Source: CAD feature listing. Evaluate the final solid. Frame: model axes, mm. Face numbers are marked on the shaded views. Give positions to 0.01 mm unless a question says otherwise; leave off trailing zeros. Loops run counter-clockwise (first coordinate to the right, second up) from the corner with the lowest first, then second, coordinate; pieces in that order, holes last.
from build123d import *

# Parameters (mm, degrees)
SKETCH_1_R          = 28
SKETCH_1_R_2        = 2.15
SKETCH_1_R_3        = 15
EXTRUDE_1_DEPTH     = 5
CUT_EXTRUDE_3_DEPTH = 1
SKETCH_5_R          = 5
CUT_EXTRUDE_5_DEPTH = 2
SKETCH_6_R          = 4.5
CUT_EXTRUDE_6_DEPTH = 1


with BuildPart() as part:
    # 草图1 → 凸台-拉伸1 (new body)
    with BuildSketch(Plane(origin=(0, 0, 0), x_dir=(1, 0, 0), z_dir=(0, 1, 0))):
        Circle(SKETCH_1_R)
        with Locations((13.980630511, -16.661466638)):
            Circle(SKETCH_1_R_2, mode=Mode.SUBTRACT)
        with Locations((13.980630511, 16.661466638)):
            Circle(SKETCH_1_R_2, mode=Mode.SUBTRACT)
        with Locations((21.75, 0)):
            Circle(SKETCH_1_R_2, mode=Mode.SUBTRACT)
        with Locations((-13.980630511, -16.661466638)):
            Circle(SKETCH_1_R_2, mode=Mode.SUBTRACT)
        with Locations((-21.75, 0)):
            Circle(SKETCH_1_R_2, mode=Mode.SUBTRACT)
        with Locations((-13.980630511, 16.661466638)):
            Circle(SKETCH_1_R_2, mode=Mode.SUBTRACT)
        Circle(SKETCH_1_R_3, mode=Mode.SUBTRACT)
    extrude(amount=EXTRUDE_1_DEPTH)

    # 草图2 → 切除-拉伸3 (cut)
    with BuildSketch(Plane(origin=(0, 0, 0), x_dir=(1, 0, 0), z_dir=(0, 1, 0))):
        with BuildLine():
            Line((3.535533906, -26.535533906), (3.535533906, -27.775888825))
            ThreePointArc((3.535533906, -27.775888825), (0, -28), (-3.535533906, -27.775888825))
            Line((-3.535533906, -27.775888825), (-3.535533906, -26.535533906))
            ThreePointArc((-3.535533906, -26.535533906), (0, -18), (3.535533906, -26.535533906))
        make_face()
    extrude(amount=CUT_EXTRUDE_3_DEPTH, mode=Mode.SUBTRACT)

    # 草图5 → 切除-拉伸5 (cut)
    with BuildSketch(Plane.XZ):
        with Locations((-13.980630511, 16.661466638)):
            Circle(SKETCH_5_R)
        with Locations((-21.75, 0)):
            Circle(SKETCH_5_R)
        with Locations((-13.980630511, -16.661466638)):
            Circle(SKETCH_5_R)
    extrude(amount=-CUT_EXTRUDE_5_DEPTH, mode=Mode.SUBTRACT)

    # 草图6 → 切除-拉伸6 (cut)
    with BuildSketch(Plane.XZ.offset(-1)):
        with Locations((0, 23)):
            Circle(SKETCH_6_R)
    extrude(amount=-CUT_EXTRUDE_6_DEPTH, mode=Mode.SUBTRACT)

    # 草图7 → 旋转1 (revolve)
    with BuildSketch(Plane(origin=(0, 0, 0), x_dir=(0, -1, 0), z_dir=(-1, 0, 0))):
        Polygon((-2, 23), (-1, 23), (-2, 27.5), align=None)
    revolve(axis=Axis((0, 2, 23), (0, -1, 0)))


solid = part.part
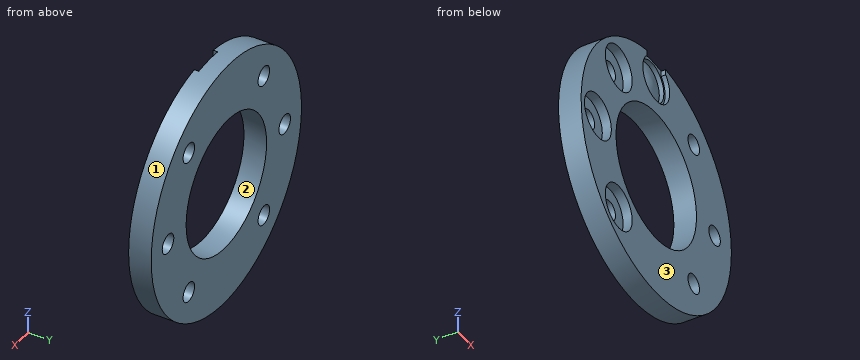
1) Cut plane C-C (y = 3.6). Return loops of the section in (x, z), and give its area (3 significant figures).
Checks:
outline: circle Ø56 at (0, 0); hole circle Ø4.3 at (-21.75, 0); hole circle Ø4.3 at (-13.98, -16.66); hole circle Ø4.3 at (-13.98, 16.66); hole circle Ø30 at (0, 0); hole circle Ø4.3 at (13.98, -16.66); hole circle Ø4.3 at (13.98, 16.66); hole circle Ø4.3 at (21.75, 0)
area: 1,670 mm2
2) Cut plane D-D (z = -11). Return loops of the section in (x, y), and give its area (3 significant figures).
Checks:
outline: (-25.75, 0) - (-10.2, 0) - (-10.2, 5) - (-25.75, 5) - close; (10.2, 0) - (25.75, 0) - (25.75, 5) - (10.2, 5) - close
area: 156 mm2
3) Ray query, probe 1 along Z at (x, y) = (-12, 3.05); probe 2 along X at (y, z) = (0.6, -4.5); probe 3 along X at (y, z) = (3.3, -16.5). Return the intervals inside material, ascending.
Checks:
probe 1: z = -25.3 to -17.5, -15.83 to -9, 9 to 15.83, 17.5 to 25.3
probe 2: x = -27.64 to -23.93, -19.57 to -14.31, 14.31 to 27.64
probe 3: x = -22.62 to -16.12, -11.84 to 11.84, 16.12 to 22.62
4) Contact query for flat-ended pins moving along their axis: P1, Ø1, axis at x = -16, y = 4, coming from the +Z side; P2, Ø3, axis at x = 21, y = 4, coming from the +Z side; P3, Ø7, axis at x = -13.98, z = -16.66, coming from the -Y side. Output: stop coordinate, or through.
Checks:
P1: stops at z = 23.32
P2: stops at z = 20.09
P3: stops at y = 2
5) Cut plane A-A (z = 0). Return loops of the section in (x, y), and give its area (3 significant figures).
Checks:
outline: (-28, 0) - (-26.75, 0) - (-26.75, 2) - (-23.9, 2) - (-23.9, 5) - (-28, 5) - close; (-19.6, 2) - (-16.75, 2) - (-16.75, 0) - (-15, 0) - (-15, 5) - (-19.6, 5) - close; (15, 0) - (19.6, 0) - (19.6, 5) - (15, 5) - close; (23.9, 0) - (28, 0) - (28, 5) - (23.9, 5) - close
area: 75.6 mm2
6) Cut plane B-B (x = -21.75). Return loops of the section in (y, z), and give its area (3 significant figures).
Checks:
outline: (0, -17.63) - (5, -17.63) - (5, -2.15) - (2, -2.15) - (2, -5) - (0, -5) - close; (0, 5) - (2, 5) - (2, 2.15) - (5, 2.15) - (5, 17.63) - (0, 17.63) - close
area: 143 mm2
7) Pull-direction query (X, two-part tool) for the marked faces 1, 2 and 3; classes: released by +X, released by -X, zero draft, split by the parting line, or undercut.
Checks:
face 1: split by the parting line
face 2: undercut
face 3: zero draft
